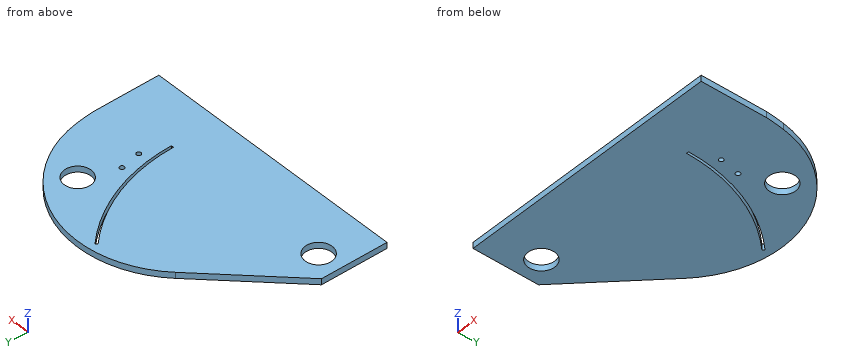
from build123d import *

# Parameters (mm, degrees)
SKETCH1_R               = 14.2748
BOSS_EXTRUDE1_DEPTH     = 6.35
CUT_EXTRUDE1_DEPTH      = 7.35
SKETCH3_R               = 14.2748
CUT_EXTRUDE2_DEPTH      = 7.35
SKETCH5_R               = 2.413
CUT_EXTRUDE3_DEPTH      = 1
CUT_EXTRUDE3_DEPTH_BACK = 7.35
FILLET1_R               = 114.3


with BuildPart() as part:
    # Sketch1 → Boss-Extrude1 (new body)
    with BuildSketch(Plane.XY):
        with BuildLine():
            Line((-25.4, -50.8), (254, -50.8))
            Line((254, -50.8), (254, 19.05))
            ThreePointArc((254, 19.05), (224.503557522, 120.320634806), (156.508042902, 200.958042902))
            Line((156.508042902, 200.958042902), (-25.4, 19.05))
            Line((-25.4, 19.05), (-25.4, -50.8))
        make_face()
        Circle(SKETCH1_R, mode=Mode.SUBTRACT)
    extrude(amount=BOSS_EXTRUDE1_DEPTH)

    # Sketch2 → Cut-Extrude1 (cut, through all)
    with BuildSketch(Plane.XY.offset(6.35)):
        with BuildLine():
            Line((127.519636919, 127.519636919), (125.723585695, 125.723585695))
            ThreePointArc((125.723585695, 125.723585695), (164.265780881, 68.041114275), (177.8, 0))
            Line((177.8, 0), (180.34, 0))
            ThreePointArc((180.34, 0), (166.612434893, 69.013130193), (127.519636919, 127.519636919))
        make_face()
    extrude(amount=-CUT_EXTRUDE1_DEPTH, mode=Mode.SUBTRACT)

    # Sketch3 → Cut-Extrude2 (cut, through all)
    with BuildSketch(Plane.XY.offset(6.35)):
        with Locations((199.741193703, 83.004946712)):
            Circle(SKETCH3_R)
    extrude(amount=-CUT_EXTRUDE2_DEPTH, mode=Mode.SUBTRACT)

    # Sketch5 → Cut-Extrude3 (cut, two sides)
    with BuildSketch(Plane.XY.offset(6.35)) as cut_extrude3_sk:
        with Locations((185.661672995, 48.015373378)):
            Circle(SKETCH5_R)
        with Locations((189.940787606, 26.424044045)):
            Circle(SKETCH5_R)
    extrude(amount=CUT_EXTRUDE3_DEPTH, mode=Mode.SUBTRACT)
    extrude(cut_extrude3_sk.sketch, amount=-CUT_EXTRUDE3_DEPTH_BACK, mode=Mode.SUBTRACT)

    # Fillet1
    fillet1_edges = [part.edges().sort_by_distance(p)[0] for p in [
        (156.508042902, 200.958042902, 3.175),
    ]]
    fillet(fillet1_edges, radius=FILLET1_R)


solid = part.part
Source: CAD feature listing. Evaluate the final solid. Frame: model axes, mm. Round coordinates to 2 decimals unless told otherwise and drop trailing zeros. Order: outer loops, then holes, each group sorted by start corner. A loop starts at its lowest first (then second) coordinate and runs counter-clockwise, first axis right, second up. Notation, with made-up numbers: (-11, 7) -> (32, 7) arc R16 ccw to (32, 38) -> close; hole circle Ø11 at (68, 32). An arc over 180 degrees is marked (long way). Answer as CSV lines item,"result".
Item 1: Line query: L1, parallel to X at y = 71, z = 3.5; L2, parallel to X at y = 87, z = 3; L3, parallel to Y at x = 146.5, z = 5.75. Output: solid intervals per line, ascending.
A:
L1,"26.55 to 163.01, 165.78 to 192.02, 207.46 to 241.8"
L2,"42.55 to 155.06, 157.97 to 186.04, 213.45 to 232.46"
L3,"-50.8 to 100.75, 105.17 to 135.59"
Item 2: Section C-C, the plane z = 5. Return loops of the section in (x, y).
A:
outline,"(-25.4, -50.8) -> (254, -50.8) -> (254, 19.05) arc R254.71 ccw to (251.69, 39.1) arc R114.3 ccw to (57.93, 102.38) -> (-25.4, 19.05) -> close; hole circle Ø28.55 at (0, 0); hole (125.72, 125.72) arc R177.8 cw to (177.8, 0) -> (180.34, 0) arc R180.34 ccw to (127.52, 127.52) -> close; hole circle Ø4.83 at (185.66, 48.02); hole circle Ø28.55 at (199.74, 83); hole circle Ø4.83 at (189.94, 26.42)"
Item 3: Section D-D, the plane x = 222. Return loops of the section in (y, z).
A:
outline,"(-50.8, 0) -> (99.87, 0) -> (99.87, 6.35) -> (-50.8, 6.35) -> close"
Item 4: Section A-A, the plane x = 0. Return loops of the section in (y, z), plus the area to 3 significant figures.
A:
outline,"(-50.8, 0) -> (-14.27, 0) -> (-14.27, 6.35) -> (-50.8, 6.35) -> close; (14.27, 0) -> (44.45, 0) -> (44.45, 6.35) -> (14.27, 6.35) -> close"
area,"424 mm²"
Item 5: Pin query (flat end, axial travel): pin 1 Ø0.8 at (x, z) = (179, 2.5) entering from +Y; pin 2 Ø1 at (y, z) = (63, 5.5) entering from +X; pin 3 Ø1 at (x, y) = (121.5, 36.5) entering from -Z; pin 4 Ø3 at (y, z) = (115.5, 3.5) entering from -X. Return the tip coordinate at first contact, or that it passes through.
A:
pin 1,"y = 128.68"
pin 2,"x = 245.46"
pin 3,"z = 0"
pin 4,"x = 71.53"
Item 6: Section B-B, the plane y = 106.5. Return loops of the section in (x, z).
A:
outline,"(62.27, 0) -> (142.37, 0) -> (142.37, 6.35) -> (62.27, 6.35) -> close; (145.53, 0) -> (215.23, 0) -> (215.23, 6.35) -> (145.53, 6.35) -> close"
